```python
from build123d import *

# Parameters (mm, degrees)
BOSS_EXTRUDE1_DEPTH = 5
CUT_EXTRUDE1_DEPTH  = 124.722915669
SKETCH3_W           = 20
SKETCH3_H           = 10
BOSS_EXTRUDE2_DEPTH = 40
SKETCH4_R           = 6.475
CUT_EXTRUDE2_DEPTH  = 137.198467549
FILLET3_R           = 2


with BuildPart() as part:
    # Sketch1 → Boss-Extrude1 (new body)
    with BuildSketch(Plane(origin=(0, 0, 0), x_dir=(1, 0, 0), z_dir=(0, 1, 0))):
        Polygon((-29.999623956, -119.926382831), (30.000376044, -119.926382831), (30.000376044, -99.926382831), (10.000376044, -99.926382831), (10.000376044, 10.073617169), (30.000376044, 10.073617169), (30.000376044, 30.073617169), (-29.999623956, 30.073617169), (-29.999623956, 10.073617169), (-9.999623956, 10.073617169), (-9.999623956, -99.926382831), (-29.999623956, -99.926382831), align=None)
    extrude(amount=BOSS_EXTRUDE1_DEPTH)

    # Sketch2 → Cut-Extrude1 (cut, through all)
    with BuildSketch(Plane(origin=(0, 5, 0), x_dir=(1, 0, 0), z_dir=(0, 1, 0))):
        with BuildLine():
            Line((-18.549247911, 18.573617169), (18.55, 18.573617169))
            ThreePointArc((18.55, 18.573617169), (19.575304833, 18.998312337), (20, 20.023617169))
            Line((20, 20.023617169), (20, 20.123617169))
            ThreePointArc((20, 20.123617169), (19.575304833, 21.148922002), (18.55, 21.573617169))
            Line((18.55, 21.573617169), (-18.549247911, 21.573617169))
            ThreePointArc((-18.549247911, 21.573617169), (-19.574552744, 21.148922002), (-19.999247911, 20.123617169))
            Line((-19.999247911, 20.123617169), (-19.999247911, 20.023617169))
            ThreePointArc((-19.999247911, 20.023617169), (-19.574552744, 18.998312337), (-18.549247911, 18.573617169))
        make_face()
        with BuildLine():
            Line((-18.549623956, -111.426382831), (18.550376044, -111.426382831))
            ThreePointArc((18.550376044, -111.426382831), (19.575680877, -111.001687663), (20.000376044, -109.976382831))
            Line((20.000376044, -109.976382831), (20.000376044, -109.876382831))
            ThreePointArc((20.000376044, -109.876382831), (19.575680877, -108.851077998), (18.550376044, -108.426382831))
            Line((18.550376044, -108.426382831), (-18.549623956, -108.426382831))
            ThreePointArc((-18.549623956, -108.426382831), (-19.574928788, -108.851077998), (-19.999623956, -109.876382831))
            Line((-19.999623956, -109.876382831), (-19.999623956, -109.976382831))
            ThreePointArc((-19.999623956, -109.976382831), (-19.574928788, -111.001687663), (-18.549623956, -111.426382831))
        make_face()
    extrude(amount=-CUT_EXTRUDE1_DEPTH, mode=Mode.SUBTRACT)

    # Sketch3 → Boss-Extrude2 (add)
    with BuildSketch(Plane(origin=(0, 5, 0), x_dir=(1, 0, 0), z_dir=(0, 1, 0))):
        with Locations((0.000376044, 0.073617169)):
            Rectangle(SKETCH3_W, SKETCH3_H)
        with Locations((0.000376044, -89.926382831)):
            Rectangle(SKETCH3_W, SKETCH3_H)
    extrude(amount=BOSS_EXTRUDE2_DEPTH)

    # Sketch4 → Cut-Extrude2 (cut, through all)
    with BuildSketch(Plane(origin=(0, 0, -5.073617169), x_dir=(-1, 0, 0), z_dir=(0, 0, -1))):
        with Locations((-0.000376044, 45)):
            Circle(SKETCH4_R)
    extrude(amount=-CUT_EXTRUDE2_DEPTH, mode=Mode.SUBTRACT)

    # Fillet3
    fillet3_edges = [part.edges().sort_by_distance(p)[0] for p in [
        (-9.999623956, 45, 89.926382831),
        (10.000376044, 45, 89.926382831),
        (0.000376044, 5, 84.926382831),
        (0.000376044, 5, 94.926382831),
        (-29.999623956, 2.5, -10.073617169),
        (-29.999623956, 2.5, -30.073617169),
        (30.000376044, 2.5, -30.073617169),
        (30.000376044, 2.5, -10.073617169),
        (10.000376044, 2.5, -10.073617169),
        (10.000376044, 2.5, 99.926382831),
        (30.000376044, 2.5, 99.926382831),
        (30.000376044, 2.5, 119.926382831),
        (-29.999623956, 2.5, 119.926382831),
        (-29.999623956, 2.5, 99.926382831),
        (-9.999623956, 2.5, 99.926382831),
        (0.000376044, 5, -5.073617169),
        (0.000376044, 5, 4.926382831),
        (10.000376044, 45, -0.073617169),
        (-9.999623956, 45, -0.073617169),
    ]]
    fillet(fillet3_edges, radius=FILLET3_R)


solid = part.part
```
Read the model definition and answer for the solid it produces. Units are mm, in the model's axes. A direction names the side the tool comes from. Round coordinates to 2 decimals unless told otherwise and drop trailing zeros. Write each loop counter-clockwise with the first axis right and the second up, starting at its lowest first coordinate (ties: lowest second). Pieces come first, ordered by that corner, then holes. Notation, with made-up numbers: (89.5, 6) - (103.5, 6) arc R27 cw to (103.5, 29) - close; hole circle Ø6 at (88.5, -33). An arc over 180 degrees is marked (long way). One line per item, written item: value.
Q1. Find section D-D (x = 4.5). Determine the outline of the cut face in (y, z), and give its area (3 significant figures).
The answers:
outline: (0, -30.07) - (5, -30.07) - (5, -21.57) - (0, -21.57) - close; (0, -18.57) - (5, -18.57) - (5, -7.07) arc R2 cw to (7, -5.07) - (40.34, -5.07) - (40.34, 4.93) - (7, 4.93) arc R2 cw to (5, 6.93) - (5, 82.93) arc R2 cw to (7, 84.93) - (40.34, 84.93) - (40.34, 94.93) - (7, 94.93) arc R2 cw to (5, 96.93) - (5, 108.43) - (0, 108.43) - close; (0, 111.43) - (5, 111.43) - (5, 119.93) - (0, 119.93) - close
area: 1,430 mm2
Q2. Find section A-A (x = 16). Determine the outline of the cut face in (y, z), and give its area (3 significant figures).
The answers:
outline: (0, -30.07) - (5, -30.07) - (5, -21.57) - (0, -21.57) - close; (0, -18.57) - (5, -18.57) - (5, -10.07) - (0, -10.07) - close; (0, 99.93) - (5, 99.93) - (5, 108.43) - (0, 108.43) - close; (0, 111.43) - (5, 111.43) - (5, 119.93) - (0, 119.93) - close
area: 170 mm2
Q3. For a pull along X with two mould halves and no side action, classify faces 5 (the flat face through (0, 26, -5.074)), 6 (the flat face through (-30, 2, -20)), 7 (the cylindrical face through (0.143, 38.527, 89.856)) as pulls with the +X half, pulls with the -X half, needs draft (parallel to the pull), parting line crosses it, or undercut.
The answers:
face 5: needs draft
face 6: pulls with the -X half
face 7: undercut
Q4. Straight lines are drawn through the part: line 1 (Z direction, x = 4, y = 38); line 2 (Z direction, x = 13, y = 4.5); line 3 (X direction, y = 31, z = 3). For each, find the intervals that lie inside material, in ascending order. Write a range as from..to.
The answers:
line 1: z = -5.07..4.93, 84.93..94.93
line 2: z = -30.07..-21.57, -18.57..-10.07, 99.93..108.43, 111.43..119.93
line 3: x = -10..10
Q5. Find section C-C (z = 88). Determine the outline of the cut face in (x, y) (3 decimals), and give its area (3 significant figures).
The answers:
outline: (-10, 0) - (10, 0) - (10, 43) arc R2 ccw to (8, 45) - (6.475, 45) arc R6.475 cw to (-6.475, 45) - (-8, 45) arc R2 ccw to (-10, 43) - close
area: 832 mm2
Q6. Find section B-B (y = 28.5). Determine the outline of the cut face in (x, z).
The answers:
outline: (-10, -5.07) - (10, -5.07) - (10, 4.93) - (-10, 4.93) - close; (-10, 84.93) - (10, 84.93) - (10, 94.93) - (-10, 94.93) - close
Q7. Each of these flat-tipped pins is pushed along its axis until it touches: P1, Ø16, axis at x = 3, z = 61, coming from the +Y side; P2, Ø1.5, axis at x = -8.5, z = 6, coming from the +Y side; P3, Ø10, axis at x = -2.5, y = 31, coming from the +Z side. Where does it stop, or does it pass through?
The answers:
P1: stops at y = 5
P2: stops at y = 5.91
P3: stops at z = 94.93
Q8. Which of the six approach directions +Z, -Z, +X, -X, +Y, -Y give full straight-line access (tool end or side, diameter ignored) to faces 1 (the flat face through (0, 5, -16)), 2 (the flat face through (20, 2, 99.926)), 3 (the flat face through (-19, 2, -10.074)), 4 (the flat face through (0, 26, 4.926))?
The answers:
face 1: -Z, +X, -X, +Y
face 2: +X, +Y, -Y
face 3: -X, +Y, -Y
face 4: +X, -X, +Y
